Can you work these out from the model? Positions are in its coordinate system, mm. A direction names the side the tool comes from. Give positions to 0.01 mm unless a question says otherwise; leave off trailing zeros. Order: outer loops, then holes, each group sorted by start corner. A loop starts at its lowest first (then second) coordinate and runs counter-clockwise, first axis right, second up. Notation, with made-up numbers: (-36, 13.5) - (2, 13.5) arc R16 cw to (2, 22.5) - close; hole circle Ø2 at (77.25, -28.5). An arc over 180 degrees is marked (long way). Answer as a JSON object with one key per item and string values.
```python
from build123d import *

# Parameters (mm, degrees)
SKETCH_1_R          = 1.5
EXTRUDE_1_DEPTH     = 12
FILLET_1_R          = 1.5
EXTRUDE_2_DEPTH     = 12
SKETCH_3_W          = 12
SKETCH_3_H          = 7
EXTRUDE_4_DEPTH     = 3
FILLET_3_R          = 5
SKETCH_4_R          = 1.5
CUT_EXTRUDE_1_DEPTH = 35.467375879
FILLET_4_R          = 10
FILLET_5_R          = 10


with BuildPart() as part:
    # 草图1 → 凸台-拉伸1 (new body)
    with BuildSketch(Plane.XY):
        with BuildLine():
            Line((-4, 7), (-4, 17))
            Line((-4, 17), (3, 17))
            Line((3, 17), (3, 20))
            Line((3, 20), (-9, 30))
            Line((-9, 30), (-12, 30))
            Line((-12, 30), (-12, 7))
            ThreePointArc((-12, 7), (-8.222207225, -1.325379685), (0.530973451, -3.96460177))
            ThreePointArc((0.530973451, -3.96460177), (3.96460177, 0.530973451), (-0.530973451, 3.96460177))
            ThreePointArc((-0.530973451, 3.96460177), (-2.954170362, 4.695233872), (-4, 7))
        make_face()
        Circle(SKETCH_1_R, mode=Mode.SUBTRACT)
        with Locations((-8, 12.68857754)):
            Circle(SKETCH_1_R, mode=Mode.SUBTRACT)
    extrude(amount=EXTRUDE_1_DEPTH)

    # 圆角1
    fillet_1_edges = [part.edges().sort_by_distance(p)[0] for p in [
        (-4, 17, 6),
    ]]
    fillet(fillet_1_edges, radius=FILLET_1_R)

    # 草图2 → 凸台-拉伸2 (add)
    with BuildSketch(Plane(origin=(0, 0, 0), x_dir=(-1, 0, 0), z_dir=(0, 0, -1))):
        Polygon((-4, 0), (-4, -9), (0, -9), (0, -4.022703843), align=None)
    extrude(amount=-EXTRUDE_2_DEPTH)

    # 草图3 → 凸台-拉伸4 (add)
    with BuildSketch(Plane.ZY):
        with Locations((6, -5.5)):
            Rectangle(SKETCH_3_W, SKETCH_3_H)
    extrude(amount=EXTRUDE_4_DEPTH)

    # 圆角3
    fillet_3_edges = [part.edges().sort_by_distance(p)[0] for p in [
        (4, -9, 6),
    ]]
    fillet(fillet_3_edges, radius=FILLET_3_R)

    # 草图4 → 切除-拉伸1 (cut, through all)
    with BuildSketch(Plane(origin=(0, 0, 0), x_dir=(-1, 0, 0), z_dir=(0, 0, -1))):
        with Locations((4.5, -3.473180033)):
            Circle(SKETCH_4_R)
    extrude(amount=-CUT_EXTRUDE_1_DEPTH, mode=Mode.SUBTRACT)

    # 圆角4
    fillet_4_edges = [part.edges().sort_by_distance(p)[0] for p in [
        (-5.884075597, -2.894963169, 6),
    ]]
    fillet(fillet_4_edges, radius=FILLET_4_R)

    # 圆角5
    # the kernel refuses this fillet: 10 mm, written as the material it takes off along each edge
    with BuildSketch(Plane(origin=(-3.050425983, -3.858842021, 12.906172426), x_dir=(0.1384631917279628, 0.990367580515692, 0), z_dir=(0, 0, -1))) as fillet_5_piece_1:
        with BuildLine():
            CenterArc((1.570698872, 9.926740679), FILLET_5_R, 260.94796551, 2.112432444)
            ThreePointArc((-0.002615053, 0.051282042), (-0.001337281, 0.025639504), (0, 0))
            ThreePointArc((0, 0), (0.181234485, 0.010988898), (0.36246897, 0))
        make_face()
    extrude(amount=13.812344852, mode=Mode.SUBTRACT)


solid = part.part
```
Q1. We'd pull the mould along X, two halves only. Please class faces 1 (the face through (-1.5, 0.07, 5.92)), 2 (the face through (-6, 10, 0)), 3 (the face through (3, 18, 6)), 4 (the face through (-9.5, 12.75, 5.92)): released by +X, released by -X, zero draft, split by the parting line, or undercut.
Recorded:
{"face 1": "undercut", "face 2": "zero draft", "face 3": "released by +X", "face 4": "undercut"}
Q2. I'm going to push flat-ended pins straight in: pin 1 Ø3.5 at (y, z) = (18.5, 5.5) entering from +X; pin 2 Ø7 at (y, z) = (10.5, 5.5) entering from +X; pin 3 Ø2.5 at (y, z) = (-6, 4.5) entering from -X. Where does each tip first touch, or does it pass through?
Recorded:
{"pin 1": "stops at x = 3", "pin 2": "stops at x = -4", "pin 3": "stops at x = -3"}
Q3. I need wall thicknesses on L1, parallel to Y at x = 0, z = 4.5; L2, parallel to Y at x = -1.25, z = 7.25; L3, parallel to X at y = -3.5, z = 2.5. Which ranges of each line are inside material? Lowest first, please.
Recorded:
{"L1": "y = -8.9 to -1.5, 1.5 to 4, 17 to 22.5", "L2": "y = -9 to -0.83, 0.83 to 3.95, 17 to 23.54", "L3": "x = -3 to 4"}
Q4. If we section it at A-A, the plane x = 0: Please give me the cut outline in (y, z).
Recorded:
{"outline": "(-8.9, 0) - (-1.5, 0) - (-1.5, 12) - (-8.9, 12) - close; (1.5, 0) - (4, 0) - (4, 12) - (1.5, 12) - close; (17, 0) - (22.5, 0) - (22.5, 12) - (17, 12) - close"}
Q5. If we section it at B-B, the plane z = 4.75: Count the separate pieces of the cut face and the enclosed holes in it, then the cut area to 3 significant figures.
Recorded:
{"separate pieces": "1", "enclosed holes": "2", "area": "344 mm^2"}
Q6. Which directions (+Z, -Z, +X, -X, +Y, -Y) give clear straight access to the entire face, cutting with the end or side of a thin tool? Please do faces 5 (the face through (-3, -6, 6)), 6 (the face through (-4, 11, 6)), 7 (the face through (-2.927, 4.671, 5.916)), 8 (the face through (-3, 25, 6)), 9 (the face through (4, -2, 6)).
Recorded:
{"face 5": "+Z, -Z, -X, -Y", "face 6": "+Z, -Z, +X", "face 7": "+Z, -Z", "face 8": "+Z, -Z, +X, +Y", "face 9": "+Z, -Z, +X, +Y, -Y"}
Q7. If we section it at C-C, the plane y = -3: Please give me the cut outline in (x, z).
Recorded:
{"outline": "(-3.08, 0) - (4, 0) - (4, 12) - (-3.08, 12) - close"}
